Part print with two shaded views. Sizes in mm from the minimum x, y, z corner. A direction names the side the tool comes from. Give positions to 0.01 mm unless a question says otherwise; leave off trailing zeros. Order: outer loops, then holes, each group sorted by start corner. A loop starts at its lowest first (then second) coordinate and runs counter-clockwise, first axis right, second up. Notation, with made-up numbers: M -9.75,-25 L 46.25,-25 A13 cw 46.25,-5 Z; hole C 44,34 d11. An arc over 180 degrees is marked long. Return JSON: item names as keys, results as strings. Group by question number.
1. 3-axis set-ups, long thin cutter, end or side, ignore diameter. For the marked faces 5, 6 and 7: which of +Z, -Z, +X, -X, +Y, -Y reach the whole face in a straight line?
2. Wall check: probe 1 along Y at (x, z) = (6.65, 18.9); probe 2 along Z at (x, y) = (6.25, 14); probe 3 along Y at (x, z) = (6.65, 17.75). Give the ranges that are in metal, low to high. Write a range as [from, to].
3. Slice it at D-D on y = 11.75. List the corners of the cut face in (x, z).
4. Slice it at A-A on x = 6.65. Give the number of separate pieces and of enclosed holes in the cut face.
5. Pin check, flat tips, straight feed: pin 1 (5.5 mm diameter, centred on x = 5.5, y = 11, fed in from -Z); pin 2 (1 mm diameter, centred on x = 6, y = 6.5, fed in from +Z); pin 3 (2 mm diameter, centred on x = 11, y = 7.5, fed in from -Z) (1 decimal); pin 4 (1.5 mm diameter, centred on x = 2, y = 6.5, fed in from -Z). Stop position of each tip, or through.
6. Two-plate mould, pull along Z, no slides. Class the marked faces 1, 2, 3 and 4: released by +Z, released by -Z, zero draft, split by the parting line, or undercut.
7. Slice it at B-B on y = 9.25. List the corners of the cut face in (x, z).
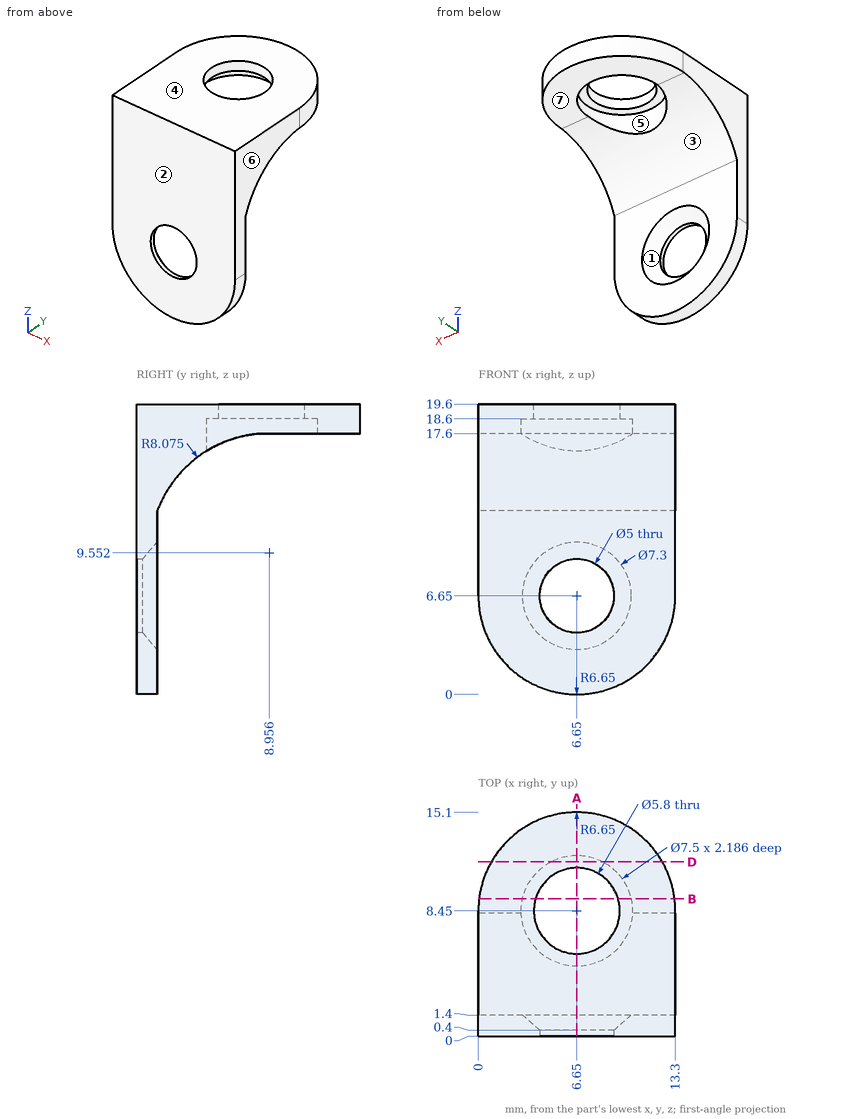
Result:
{
 "1": {"face 5": "-Z", "face 6": "+Z, -Z, +X, +Y, -Y", "face 7": "-Z, +X, -X, +Y"},
 "2": {"probe 1": "y = [0, 5.55], [11.35, 15.1]", "probe 2": "z = [17.6, 19.6]", "probe 3": "y = [0, 4.7], [12.2, 15.1]"},
 "3": {"outline": "M 0.88,17.6 L 4.87,17.6 L 4.87,18.6 L 8.43,18.6 L 8.43,17.6 L 12.42,17.6 L 12.42,19.6 L 0.88,19.6 Z"},
 "4": {"separate pieces": "3", "enclosed holes": "0"},
 "5": {"pin 1": "stops at z = 17.6", "pin 2": "passes through", "pin 3": "stops at z = 17.2", "pin 4": "stops at z = 16.96"},
 "6": {"face 1": "undercut", "face 2": "zero draft", "face 3": "released by -Z", "face 4": "released by +Z"},
 "7": {"outline": "M 0.05,17.6 L 2.99,17.6 L 2.99,18.6 L 3.86,18.6 L 3.86,19.6 L 0.05,19.6 Z; M 9.44,18.6 L 10.31,18.6 L 10.31,17.6 L 13.25,17.6 L 13.25,19.6 L 9.44,19.6 Z"}
}
